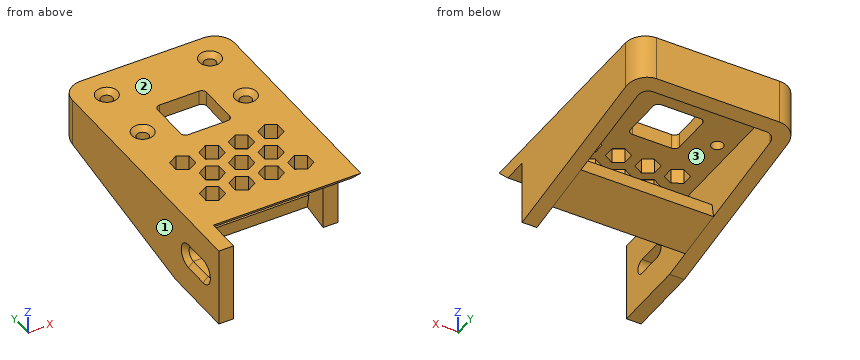
from build123d import *

# Parameters (mm, degrees)
SKETCH1_W                                       = 33
SKETCH1_H                                       = 40
BOSS_EXTRUDE1_DEPTH                             = 3
SKETCH2_W                                       = 33
SKETCH2_H                                       = 40
SKETCH2_W_2                                     = 27
SKETCH2_H_2                                     = 34
BOSS_EXTRUDE2_DEPTH                             = 3
SKETCH3_W                                       = 10
SKETCH3_H                                       = 10
CUT_EXTRUDE1_DEPTH                              = 3
CSK_FOR_M2_FLAT_HEAD_MACHINE_SCREW1_D           = 2.4
CSK_FOR_M2_FLAT_HEAD_MACHINE_SCREW1_DEPTH       = 5
CSK_FOR_M2_FLAT_HEAD_MACHINE_SCREW1_CSINK_D     = 4.4
CSK_FOR_M2_FLAT_HEAD_MACHINE_SCREW1_CSINK_ANGLE = 90
CSK_FOR_M2_FLAT_HEAD_MACHINE_SCREW1_TIP         = 0.721032743
BOSS_EXTRUDE4_DEPTH                             = 3
FILLET1_R                                       = 1
BOSS_EXTRUDE5_REACH                             = 29.809
SKETCH15_W                                      = 27
SKETCH15_H                                      = 3
SKETCH16_W                                      = 27
SKETCH16_H                                      = 3
CUT_EXTRUDE6_DEPTH                              = 3
SKETCH18_W                                      = 27
SKETCH18_H                                      = 10
BOSS_EXTRUDE6_DEPTH                             = 3
FILLET2_R                                       = 4
FILLET3_R                                       = 2
SKETCH21_W                                      = 16.053079228
SKETCH21_H                                      = 15
BOSS_EXTRUDE7_DEPTH                             = 3
CUT_EXTRUDE10_DEPTH                             = 10
SKETCH23_W                                      = 30
SKETCH23_H                                      = 8
BOSS_EXTRUDE8_DEPTH                             = 3
CHAMFER5_SIZE                                   = 3
CHAMFER6_SIZE                                   = 1
CUT_EXTRUDE12_DEPTH                             = 10


with BuildPart() as part:
    # Sketch1 → Boss-Extrude1 (new body)
    with BuildSketch(Plane.XY):
        Rectangle(SKETCH1_W, SKETCH1_H)
    extrude(amount=-BOSS_EXTRUDE1_DEPTH)

    # Sketch2 → Boss-Extrude2 (add)
    with BuildSketch(Plane(origin=(0, 0, -3), x_dir=(-1, 0, 0), z_dir=(0, 0, -1))):
        Rectangle(SKETCH2_W, SKETCH2_H)
        Rectangle(SKETCH2_W_2, SKETCH2_H_2, mode=Mode.SUBTRACT)
    extrude(amount=BOSS_EXTRUDE2_DEPTH)

    # Sketch3 → Cut-Extrude1 (cut)
    with BuildSketch(Plane.XY):
        with Locations((0, 2)):
            Rectangle(SKETCH3_W, SKETCH3_H)
    extrude(amount=-CUT_EXTRUDE1_DEPTH, mode=Mode.SUBTRACT)

    # CSK for M2 Flat Head Machine Screw1
    with Locations(Plane.XY):
        with Locations((10.5, 1.75), (10.5, 14.25), (-10.5, 1.75), (-10.5, 14.25)):
            CounterSinkHole(CSK_FOR_M2_FLAT_HEAD_MACHINE_SCREW1_D / 2, CSK_FOR_M2_FLAT_HEAD_MACHINE_SCREW1_CSINK_D / 2, depth=CSK_FOR_M2_FLAT_HEAD_MACHINE_SCREW1_DEPTH, counter_sink_angle=CSK_FOR_M2_FLAT_HEAD_MACHINE_SCREW1_CSINK_ANGLE)
            with Locations((0, 0, -(CSK_FOR_M2_FLAT_HEAD_MACHINE_SCREW1_DEPTH + CSK_FOR_M2_FLAT_HEAD_MACHINE_SCREW1_TIP / 2))):  # 118° drill point
                Cone(0, CSK_FOR_M2_FLAT_HEAD_MACHINE_SCREW1_D / 2, CSK_FOR_M2_FLAT_HEAD_MACHINE_SCREW1_TIP, mode=Mode.SUBTRACT)

    # Sketch11 → Boss-Extrude4 (add)
    with BuildSketch(Plane.ZY.offset(16.5)):
        Polygon((-6, 20), (-9, 20), (-16.053079228, -20), (-6, -20), align=None)
    boss_extrude4 = extrude(amount=-BOSS_EXTRUDE4_DEPTH)

    # Mirror1: Boss-Extrude4 across plane
    add(boss_extrude4.mirror(Plane(origin=(0, 0, 0), x_dir=(0, 0, 1), z_dir=(1, 0, 0))))

    # Fillet1
    fillet1_edges = [part.edges().sort_by_distance(p)[0] for p in [
        (5, 7, -1.5),
        (5, -3, -1.5),
        (-5, -3, -1.5),
        (-5, 7, -1.5),
    ]]
    fillet(fillet1_edges, radius=FILLET1_R)

    # Boss-Extrude5: up to this face of the body (flat: up to its plane)
    boss_extrude5_end = Plane(part.part.faces().sort_by_distance((15, 0, -12.526539614))[0])
    # Sketch15 → Boss-Extrude5 (add, up to the picked face)
    with BuildSketch(Plane(origin=(0, 0, -6), x_dir=(-1, 0, 0), z_dir=(0, 0, -1)), mode=Mode.PRIVATE) as boss_extrude5_sk1:
        with Locations((0, 18.5)):
            Rectangle(SKETCH15_W, SKETCH15_H)
    boss_extrude5_tool1 = split(extrude(boss_extrude5_sk1.sketch, amount=BOSS_EXTRUDE5_REACH, mode=Mode.PRIVATE), bisect_by=boss_extrude5_end, keep=Keep.BOTH, mode=Mode.PRIVATE)
    add(boss_extrude5_tool1.solids().sort_by(Axis((0, 18.5, -6), (0, 0, -1)))[0])

    # Sketch16 → Cut-Extrude6 (cut)
    with BuildSketch(Plane.XZ.offset(20)):
        with Locations((0, -4.5)):
            Rectangle(SKETCH16_W, SKETCH16_H)
    extrude(amount=-CUT_EXTRUDE6_DEPTH, mode=Mode.SUBTRACT)

    # Sketch18 → Boss-Extrude6 (add)
    with BuildSketch(Plane(origin=(0, 2.142164437, -12.148818227), x_dir=(-1, 0, 0), z_dir=(0, 0.17364817766692342, -0.9848077530122092))):
        with Locations((0, -11.912958374)):
            Rectangle(SKETCH18_W, SKETCH18_H)
    extrude(amount=-BOSS_EXTRUDE6_DEPTH)

    # Fillet2
    fillet2_edges = [part.edges().sort_by_distance(p)[0] for p in [
        (-16.5, 20, -4.5),
        (16.5, 20, -4.5),
    ]]
    fillet(fillet2_edges, radius=FILLET2_R)

    # Fillet3
    fillet3_edges = [part.edges().sort_by_distance(p)[0] for p in [
        (-13.5, 17, -6.264490471),
        (13.5, 17, -6.264490471),
    ]]
    fillet(fillet3_edges, radius=FILLET3_R)

    # Sketch21 → Boss-Extrude7 (add)
    with BuildSketch(Plane.ZY.offset(16.5)):
        with Locations((-8.026539614, -27.5)):
            Rectangle(SKETCH21_W, SKETCH21_H)
    extrude(amount=-BOSS_EXTRUDE7_DEPTH)

    # Sketch22 → Cut-Extrude10 (cut)
    with BuildSketch(Plane.ZY.offset(16.5)):
        with BuildLine():
            Line((-9.526539614, -29.555), (-9.526539614, -24.445))
            ThreePointArc((-9.526539614, -24.445), (-8.026539614, -22.945), (-6.526539614, -24.445))
            Line((-6.526539614, -24.445), (-6.526539614, -29.555))
            ThreePointArc((-6.526539614, -29.555), (-8.026539614, -31.055), (-9.526539614, -29.555))
        make_face()
    extrude(amount=-CUT_EXTRUDE10_DEPTH, mode=Mode.SUBTRACT)

    # Sketch23 → Boss-Extrude8 (add)
    with BuildSketch(Plane.XY):
        with Locations((1.5, -24)):
            Rectangle(SKETCH23_W, SKETCH23_H)
    extrude(amount=-BOSS_EXTRUDE8_DEPTH)

    # Chamfer5
    chamfer5_edges = [part.edges().sort_by_distance(p)[0] for p in [
        (1.5, -28, -3),
    ]]
    chamfer(chamfer5_edges, length=CHAMFER5_SIZE - 0.0001)  # a hair under: the kernel refuses the full size

    # Chamfer6
    chamfer6_edges = [part.edges().sort_by_distance(p)[0] for p in [
        (-16.5, -31.055, -8.026539614),
        (-16.5, -27, -6.526539614),
        (-16.5, -22.945, -8.026539614),
        (-16.5, -27, -9.526539614),
    ]]
    chamfer(chamfer6_edges, length=CHAMFER6_SIZE)

    # Sketch25 → Cut-Extrude12 (cut)
    with BuildSketch(Plane.XY):
        Polygon((-1, -8.414816681), (-3, -7.260116142), (-5, -8.414816681), (-5, -10.724217758), (-3, -11.878918296), (-1, -10.724217758), align=None)
        Polygon((-7, -8.414816681), (-9, -7.260116142), (-11, -8.414816681), (-11, -10.724217758), (-9, -11.878918296), (-7, -10.724217758), align=None)
        Polygon((1, -10.724217758), (1, -8.414816681), (3, -7.260116142), (5, -8.414816681), (5, -10.724217758), (3, -11.878918296), align=None)
        Polygon((7, -10.724217758), (7, -8.414816681), (9, -7.260116142), (11, -8.414816681), (11, -10.724217758), (9, -11.878918296), align=None)
        Polygon((0, -12.456268565), (-2, -13.610969104), (-2, -15.92037018), (0, -17.075070719), (2, -15.92037018), (2, -13.610969104), align=None)
        Polygon((-6, -12.456268565), (-8, -13.610969104), (-8, -15.92037018), (-6, -17.075070719), (-4, -15.92037018), (-4, -13.610969104), align=None)
        Polygon((6, -12.456268565), (4, -13.610969104), (4, -15.92037018), (6, -17.075070719), (8, -15.92037018), (8, -13.610969104), align=None)
        Polygon((1, -21.116522603), (3, -22.271223141), (5, -21.116522603), (5, -18.807121526), (3, -17.652420988), (1, -18.807121526), align=None)
        Polygon((7, -21.116522603), (9, -22.271223141), (11, -21.116522603), (11, -18.807121526), (9, -17.652420988), (7, -18.807121526), align=None)
        Polygon((-1, -18.807121526), (-1, -21.116522603), (-3, -22.271223141), (-5, -21.116522603), (-5, -18.807121526), (-3, -17.652420988), align=None)
        Polygon((-7, -18.807121526), (-7, -21.116522603), (-9, -22.271223141), (-11, -21.116522603), (-11, -18.807121526), (-9, -17.652420988), align=None)
    extrude(amount=-CUT_EXTRUDE12_DEPTH, mode=Mode.SUBTRACT)


solid = part.part
The model under review builds one solid part; all positions refer to its coordinate system, in mm. Face numbers are marked on the shaded views. Round coordinates to 2 decimals unless told otherwise and drop trailing zeros. Loops run counter-clockwise (first coordinate to the right, second up) from the corner with the lowest first, then second, coordinate; pieces in that order, holes last. Notation, with made-up numbers: M -22.75,7.25 L 19.25,7.25 A16 ccw 19.25,19.25 Z; hole C 30,-27.5 d1. An arc over 180 degrees is marked long. Answer as CSV lines item,"result". Start each with the question number.
Item 1: Consider section B-B (y = 8). Write out the cut boundary in (x, z).
Item 2: Consider section C-C (x = -10). State how many separate pieces and enclosed holes the cut face has, then the cut area to 3 significant figures.
Item 3: Insertion check: P1, Ø5, axis at x = 4.5, y = -28, coming from the -Z side; P2, Ø1.5, axis at x = 5.5, z = -13, coming from the -Y side; P3, Ø3, axis at x = -10.5, y = 14.25, coming from the -Z side. Each pin has a flat end and moves straight along its axis. Give the tip position at first contact, or say it passes through.
Item 4: Mouldability with a two-part tool opening along Z and no side actions: class the marked faces 1, 2 and 3 as released by +Z, released by -Z, zero draft, split by the parting line, or undercut.
Item 5: Wall thickness on line 1 (X direction, y = 14.25, z = -2.5); line 2 (X direction, y = 1.75, z = -2.45); line 3 (Y direction, x = 10.5, z = -2.2): over which ranges is each line inside the solid? List them lowest first. Write a range as [from, to].
Item 6: Consider section A-A (y = 1.75). Write out the cut boundary in (x, z).
Answer:
1,outline,"M -16.5,-11.12 L -13.5,-11.12 L -13.5,-3 L 13.5,-3 L 13.5,-11.12 L 16.5,-11.12 L 16.5,0 L -16.5,0 Z"
2,separate pieces,"6"
2,enclosed holes,"0"
2,area,"152 mm^2"
3,P1,"stops at z = -2.5"
3,P2,"stops at y = -15.01"
3,P3,"stops at z = -3"
4,face 1,"zero draft"
4,face 2,"released by +Z"
4,face 3,"undercut"
5,line 1,"x = [-16.5, -11.7], [-9.3, 9.3], [11.7, 16.5]"
5,line 2,"x = [-16.5, -11.7], [-9.3, -5], [5, 9.3], [11.7, 16.5]"
5,line 3,"y = [-25.8, -21.41], [-18.52, -11.01], [-8.13, 0.55], [2.95, 13.05], [15.45, 20]"
6,outline,"M -16.5,-12.22 L -13.5,-12.22 L -13.5,-3 L -11.7,-3 L -11.7,-1 L -12.7,0 L -16.5,0 Z; M -9.3,-3 L -5,-3 L -5,0 L -8.3,0 L -9.3,-1 Z; M 5,-3 L 9.3,-3 L 9.3,-1 L 8.3,0 L 5,0 Z; M 11.7,-3 L 13.5,-3 L 13.5,-12.22 L 16.5,-12.22 L 16.5,0 L 12.7,0 L 11.7,-1 Z"
